The listing builds one solid part. Answer for the finished solid, in the listing's coordinates (mm). A direction names the side the tool comes from. Coordinates: 2 decimals unless noted, no trailing zeros. Order: outer loops, then holes, each group sorted by start corner. A loop starts at its lowest first (then second) coordinate and runs counter-clockwise, first axis right, second up.
```python
from build123d import *

# Parameters (mm, degrees)
SKETCH1_W           = 26
SKETCH1_H           = 39
BOSS_EXTRUDE1_DEPTH = 10
SKETCH2_W           = 26
SKETCH2_H           = 5
BOSS_EXTRUDE2_DEPTH = 25
CUT_EXTRUDE1_REACH  = 71.8
CHAMFER1_SIZE       = 2
SKETCH4_W           = 54
SKETCH4_H           = 8
BOSS_EXTRUDE3_DEPTH = 9
CUT_EXTRUDE2_REACH  = 71.541
SKETCH5_R           = 2.15
SKETCH6_R           = 3.5
CUT_EXTRUDE3_DEPTH  = 5
CHAMFER3_SIZE       = 3
CUT_EXTRUDE5_DEPTH  = 1
CUT_EXTRUDE6_DEPTH  = 4
CUT_EXTRUDE7_REACH  = 71.8
SKETCH12_R          = 1.65
SKETCH14_W          = 12
SKETCH14_H          = 12
CUT_EXTRUDE9_DEPTH  = 7
SKETCH15_W          = 37.46707609
SKETCH15_H          = 12.719450185
CUT_EXTRUDE10_DEPTH = 89.977525252
SKETCH16_W          = 5
SKETCH16_H          = 12
CUT_EXTRUDE11_DEPTH = 7


with BuildPart() as part:
    # Sketch1 → Boss-Extrude1 (new body)
    with BuildSketch(Plane(origin=(0, 0, 0), x_dir=(1, 0, 0), z_dir=(0, 1, 0))):
        with Locations((13, 19.5)):
            Rectangle(SKETCH1_W, SKETCH1_H)
    extrude(amount=BOSS_EXTRUDE1_DEPTH)

    # Sketch2 → Boss-Extrude2 (add)
    with BuildSketch(Plane(origin=(0, 0, -39), x_dir=(-1, 0, 0), z_dir=(0, 0, -1))):
        with Locations((-13, 7.5)):
            Rectangle(SKETCH2_W, SKETCH2_H)
    extrude(amount=BOSS_EXTRUDE2_DEPTH)

    # Sketch3 → Cut-Extrude1 (cut, up to next)
    with BuildSketch(Plane(origin=(0, 10, 0), x_dir=(1, 0, 0), z_dir=(0, 1, 0)), mode=Mode.PRIVATE) as cut_extrude1_sk1:
        with BuildLine():
            Line((0, 54), (0, 64))
            Line((0, 64), (10, 64))
            ThreePointArc((10, 64), (7.071067812, 56.928932188), (0, 54))
        make_face()
    cut_extrude1_tool1 = extrude(cut_extrude1_sk1.sketch, amount=-CUT_EXTRUDE1_REACH, mode=Mode.PRIVATE) & part.part
    add(cut_extrude1_tool1.solids().sort_by_distance((4.244132, 10, -59.755868))[0], mode=Mode.SUBTRACT)

    # Chamfer1
    chamfer1_edges = [part.edges().sort_by_distance(p)[0] for p in [
        (26, 10, -32),
        (18, 10, -64),
        (0, 10, -27),
        (7.071067812, 10, -56.928932188),
        (13, 10, 0),
    ]]
    chamfer(chamfer1_edges, length=CHAMFER1_SIZE)

    # Sketch4 → Boss-Extrude3 (add)
    with BuildSketch(Plane.ZY):
        with Locations((-27, 4)):
            Rectangle(SKETCH4_W, SKETCH4_H)
    extrude(amount=BOSS_EXTRUDE3_DEPTH)

    # Sketch5 → Cut-Extrude2 (cut, up to next)
    with BuildSketch(Plane(origin=(0, 8, 0), x_dir=(1, 0, 0), z_dir=(0, 1, 0)), mode=Mode.PRIVATE) as cut_extrude2_sk1:
        with Locations(Location((-4.5, 48.837478231, 0), (0, 0, 270))):
            Circle(SKETCH5_R)
    cut_extrude2_tool1 = extrude(cut_extrude2_sk1.sketch, amount=-CUT_EXTRUDE2_REACH, mode=Mode.PRIVATE) & part.part
    # Sketch5 → Cut-Extrude2 (cut, up to next)
    with BuildSketch(Plane(origin=(0, 8, 0), x_dir=(1, 0, 0), z_dir=(0, 1, 0)), mode=Mode.PRIVATE) as cut_extrude2_sk2:
        with Locations(Location((-4.5, 4.837478231, 0), (0, 0, 270))):
            Circle(SKETCH5_R)
    cut_extrude2_tool2 = extrude(cut_extrude2_sk2.sketch, amount=-CUT_EXTRUDE2_REACH, mode=Mode.PRIVATE) & part.part
    add(cut_extrude2_tool1.solids().sort_by_distance((-4.5, 8, -48.837478))[0], mode=Mode.SUBTRACT)
    add(cut_extrude2_tool2.solids().sort_by_distance((-4.5, 8, -4.837478))[0], mode=Mode.SUBTRACT)

    # Sketch6 → Cut-Extrude3 (cut)
    with BuildSketch(Plane(origin=(0, 8, 0), x_dir=(1, 0, 0), z_dir=(0, 1, 0))):
        with Locations(Location((-4.5, 48.837478231, 0), (0, 0, 270))):
            Circle(SKETCH6_R)
        with Locations(Location((-4.5, 4.837478231, 0), (0, 0, 270))):
            Circle(SKETCH6_R)
    extrude(amount=-CUT_EXTRUDE3_DEPTH, mode=Mode.SUBTRACT)

    # Chamfer3
    # the kernel refuses this chamfer: 3 mm, written as the material it takes off along each edge
    with BuildSketch(Plane(origin=(-9, 8, -61.715048964), x_dir=(-0.0274958766105862, -0.9996219169112968, 0), z_dir=(0, 0, 1))) as chamfer3_piece_1:
        Polygon((CHAMFER3_SIZE * 0.999621916911, CHAMFER3_SIZE * 0.0274958766106), (-CHAMFER3_SIZE * 0.0274958766106, CHAMFER3_SIZE * 0.999621916911), (0, 0), align=None)
    extrude(amount=69.430097928, mode=Mode.SUBTRACT)

    # Sketch10 → Cut-Extrude5 (cut)
    with BuildSketch(Plane(origin=(0, 10, 0), x_dir=(1, 0, 0), z_dir=(0, 1, 0))):
        Polygon((14.732050808, 39), (13.866025404, 40.5), (12.133974596, 40.5), (11.267949192, 39), (12.133974596, 37.5), (13.866025404, 37.5), align=None)
        Polygon((14.732050808, 43.75), (13.866025404, 45.25), (12.133974596, 45.25), (11.267949192, 43.75), (12.133974596, 42.25), (13.866025404, 42.25), align=None)
        Polygon((17.979646072, 39.875), (18.845671476, 41.375), (17.979646072, 42.875), (16.247595264, 42.875), (15.38156986, 41.375), (16.247595264, 39.875), align=None)
        Polygon((16.247595264, 35.125), (17.979646072, 35.125), (18.845671476, 36.625), (17.979646072, 38.125), (16.247595264, 38.125), (15.38156986, 36.625), align=None)
        Polygon((11.267949192, 34.25), (12.133974596, 32.75), (13.866025404, 32.75), (14.732050808, 34.25), (13.866025404, 35.75), (12.133974596, 35.75), align=None)
        Polygon((8.020353928, 38.125), (7.154328524, 36.625), (8.020353928, 35.125), (9.752404736, 35.125), (10.61843014, 36.625), (9.752404736, 38.125), align=None)
        Polygon((9.752404736, 42.875), (8.020353928, 42.875), (7.154328524, 41.375), (8.020353928, 39.875), (9.752404736, 39.875), (10.61843014, 41.375), align=None)
    extrude(amount=-CUT_EXTRUDE5_DEPTH, mode=Mode.SUBTRACT)

    # Sketch11 → Cut-Extrude6 (cut)
    with BuildSketch(Plane(origin=(0, 10, 0), x_dir=(1, 0, 0), z_dir=(0, 1, 0))):
        Polygon((6.75, 44.08771324), (4, 45.675426481), (1.25, 44.08771324), (1.25, 40.91228676), (4, 39.324573519), (6.75, 40.91228676), align=None)
        Polygon((6.75, 52.08771324), (4, 53.675426481), (1.25, 52.08771324), (1.25, 48.91228676), (4, 47.324573519), (6.75, 48.91228676), align=None)
        Polygon((21.174508901, 56.076331968), (19.521149027, 58.787371337), (16.346640126, 58.711039369), (14.825491099, 55.923668032), (16.478850973, 53.212628663), (19.653359874, 53.288960631), align=None)
    extrude(amount=-CUT_EXTRUDE6_DEPTH, mode=Mode.SUBTRACT)

    # Sketch12 → Cut-Extrude7 (cut, up to next)
    with BuildSketch(Plane(origin=(0, 10, 0), x_dir=(1, 0, 0), z_dir=(0, 1, 0)), mode=Mode.PRIVATE) as cut_extrude7_sk1:
        with Locations(Location((4, 50.5, 0), (0, 0, 270))):
            Circle(SKETCH12_R)
    cut_extrude7_tool1 = extrude(cut_extrude7_sk1.sketch, amount=-CUT_EXTRUDE7_REACH, mode=Mode.PRIVATE) & part.part
    # Sketch12 → Cut-Extrude7 (cut, up to next)
    with BuildSketch(Plane(origin=(0, 10, 0), x_dir=(1, 0, 0), z_dir=(0, 1, 0)), mode=Mode.PRIVATE) as cut_extrude7_sk2:
        with Locations(Location((4, 42.5, 0), (0, 0, 270))):
            Circle(SKETCH12_R)
    cut_extrude7_tool2 = extrude(cut_extrude7_sk2.sketch, amount=-CUT_EXTRUDE7_REACH, mode=Mode.PRIVATE) & part.part
    # Sketch12 → Cut-Extrude7 (cut, up to next)
    with BuildSketch(Plane(origin=(0, 10, 0), x_dir=(1, 0, 0), z_dir=(0, 1, 0)), mode=Mode.PRIVATE) as cut_extrude7_sk3:
        with Locations(Location((18, 56, 0), (0, 0, 270))):
            Circle(SKETCH12_R)
    cut_extrude7_tool3 = extrude(cut_extrude7_sk3.sketch, amount=-CUT_EXTRUDE7_REACH, mode=Mode.PRIVATE) & part.part
    add(cut_extrude7_tool1.solids().sort_by_distance((4, 10, -50.5))[0], mode=Mode.SUBTRACT)
    add(cut_extrude7_tool2.solids().sort_by_distance((4, 10, -42.5))[0], mode=Mode.SUBTRACT)
    add(cut_extrude7_tool3.solids().sort_by_distance((18, 10, -56))[0], mode=Mode.SUBTRACT)

    # Sketch14 → Cut-Extrude9 (cut)
    with BuildSketch(Plane.XZ):
        with Locations((18.75, -23)):
            Rectangle(SKETCH14_W, SKETCH14_H)
    extrude(amount=-CUT_EXTRUDE9_DEPTH, mode=Mode.SUBTRACT)

    # Mirror3: part across plane


with BuildPart() as part_1:
    add(part.part)
    add(part.part.mirror(Plane(origin=(26, 0, 0), x_dir=(0, 0, 1), z_dir=(1, 0, 0))))

    # Sketch15 → Cut-Extrude10 (cut, through all)
    with BuildSketch(Plane.XY):
        with Locations((7.266461955, 6.359725093)):
            Rectangle(SKETCH15_W, SKETCH15_H)
    extrude(amount=-CUT_EXTRUDE10_DEPTH, mode=Mode.SUBTRACT)

    # Sketch16 → Cut-Extrude11 (cut)
    with BuildSketch(Plane.XZ):
        with Locations((41.75, -23)):
            Rectangle(SKETCH16_W, SKETCH16_H)
    extrude(amount=-CUT_EXTRUDE11_DEPTH, mode=Mode.SUBTRACT)


solid = part_1.part
```
1) Each of these flat-tipped pins is pushed along its axis until it touches: P1, Ø3.5, axis at x = 57.5, z = -47.5, coming from the +Y side; P2, Ø6, axis at x = 54.5, z = -21, coming from the +Y side; P3, Ø5.5, axis at x = 34, z = -56, coming from the -Y side; P4, Ø2, axis at x = 48, z = -42.5, coming from the -Y side. Where does it stop, or does it pass through?
2) A cutting plane is placed at C-C, the plane z = -15.5. Write down the section's boundary in (x, y), plus the area to 4 significant figures.
3) The mould has two halves that part along X. Classify faces 1 (the flat face through (50.75, 8, -51)), 2 (the flat face through (39, 5, -51)), 3 (the cylindrical face through (44.85, 6.52, -57.01)): released by +X, released by -X, zero draft, split by the parting line, or undercut.
4) For faces 4 (the cylindrical face through (55.047, 1.521, -6.422)), 5 (the cylindrical face through (53.03, 5.54, -49.29)), 6 (the flat face through (56, 4, -54)), 7 (the flat face through (55, 8, -27)), determine the directions among +Z, -Z, +X, -X, +Y, -Y from which every point of the face is accessible in a straight line to the end or side of a thin tool.
5) A cutting plane is placed at B-B, the plane x = 56.5. Write down the section's boundary in (y, z), plus the area to 3 significant figures.
6) Straight lines are drawn through the part: probe 1 along Z at (x, y) = (56.5, 1.7); probe 2 along Z at (x, y) = (37, 3.5); probe 3 along Z at (x, y) = (29, 6). For each, find the intervals that lie inside material, in ascending order.
7) A cutting plane is placed at A-A, the plane y = 1.25. Write down the section's boundary in (x, z), plus the area to 3 significant figures.
Working result:
1. P1: stops at y = 3
1. P2: stops at y = 8.5
1. P3: stops at y = 5
1. P4: passes through
2. outline: (26, 0) - (61, 0) - (61, 5) - (58, 8) - (52, 8) - (50, 10) - (28, 10) - (26, 8) - close
2. area: 323.5 mm2
3. face 1: undercut
3. face 2: zero draft
3. face 3: released by +X
4. face 4: +Y, -Y
4. face 5: +Y
4. face 6: -Z, +X, +Y, -Y
4. face 7: +Z, -Z, +X, +Y
5. outline: (0, -54) - (8, -54) - (8, -52.34) - (3, -52.34) - (3, -50.99) - (0, -50.99) - close; (0, -46.69) - (3, -46.69) - (3, -45.34) - (8, -45.34) - (8, -8.34) - (3, -8.34) - (3, -6.99) - (0, -6.99) - close; (0, -2.69) - (3, -2.69) - (3, -1.34) - (8, -1.34) - (8, 0) - (0, 0) - close
5. area: 336 mm2
6. probe 1: z = -54 to -50.99, -46.69 to -6.99, -2.69 to 0
6. probe 2: z = -39 to -29, -17 to 0
6. probe 3: z = -64 to -29, -17 to 0
7. outline: (26, -39) - (52, -39) - (52, -54) - (61, -54) - (61, 0) - (26, 0) - close; hole (27.25, -29) - (44.25, -29) - (44.25, -17) - (27.25, -17) - close; hole circle Ø4.3 at (56.5, -48.84); hole circle Ø4.3 at (56.5, -4.84)
7. area: 1,270 mm2
